Design review of the part built by this model. Coordinates are the model's own, in mm. Coordinates: 2 decimals unless noted, no trailing zeros. Loops run counter-clockwise (first coordinate to the right, second up) from the corner with the lowest first, then second, coordinate; pieces in that order, holes last.
Q1. Add section C-C on x = 11.5. Give the boundary of the cut face in (y, z).
Q2. Add section A-A on y = 0. Give the boundary of the cut face in (x, z) (3 decimals), and give its area (3 significant figures).
Q3. Wall thickness on probe 1 along X at (y, z) = (-23, -25) (3 decimals); probe 2 along Y at (x, z) = (2.45, -6.35); probe 3 along Z at (x, y) = (10, -8.5): over which ranges is each line inside the solid? List them lowest first.
Q4. Draft analysis for pull direction Z (two halves, no side actions). For faces 1 (the face through (7.871, 22.534, 11.721)), 2 (the face through (3.175, -7.8, -24.5)), 3 (the face through (1.565, 19.863, -19.846)), state which applies: released by +Z, released by -Z, zero draft, split by the parting line, or undercut.
Q5. For P1, Ø3, axis at y = -28.575, z = -6.35, coming from the +X side; P2, Ø4, axis at y = 8.79, z = -27.92, coming from the +X side (3 decimals); P3, Ø2, axis at x = 5.5, z = 20, coming from the -Y side; P4, Ø1.5, axis at x = 5, y = -11, coming from the +Z side, all flat-tipped, find the tip position at first contact; note any pin that passes through.
```python
from build123d import *

# Parameters (mm, degrees)
SKETCH2_R           = 37.5
SKETCH2_R_2         = 1.7272
SKETCH2_R_3         = 22.86
BOSS_EXTRUDE1_DEPTH = 3.175
SKETCH3_R           = 25.4
SKETCH3_R_2         = 22.86
BOSS_EXTRUDE2_DEPTH = 9.525


with BuildPart() as part:
    # Sketch2 → Boss-Extrude1 (new body)
    with BuildSketch(Plane(origin=(0, 0, 0), x_dir=(0, 0, -1), z_dir=(1, 0, 0))):
        Circle(SKETCH2_R)
        with Locations((27.921675913, 8.788238686)):
            Circle(SKETCH2_R_2, mode=Mode.SUBTRACT)
        with Locations((21.571675913, 19.786761314)):
            Circle(SKETCH2_R_2, mode=Mode.SUBTRACT)
        with Locations((-21.571675913, 19.786761314)):
            Circle(SKETCH2_R_2, mode=Mode.SUBTRACT)
        with Locations((-27.921675913, 8.788238686)):
            Circle(SKETCH2_R_2, mode=Mode.SUBTRACT)
        with Locations((-6.35, -28.575)):
            Circle(SKETCH2_R_2, mode=Mode.SUBTRACT)
        with Locations((6.35, -28.575)):
            Circle(SKETCH2_R_2, mode=Mode.SUBTRACT)
        Circle(SKETCH2_R_3, mode=Mode.SUBTRACT)
    extrude(amount=BOSS_EXTRUDE1_DEPTH)

    # Sketch3 → Boss-Extrude2 (add)
    with BuildSketch(Plane(origin=(3.175, 0, 0), x_dir=(0, 0, -1), z_dir=(1, 0, 0))):
        with Locations(Location((0, 0, 0), (0, 0, 180))):
            Circle(SKETCH3_R)
        Circle(SKETCH3_R_2, mode=Mode.SUBTRACT)
    extrude(amount=BOSS_EXTRUDE2_DEPTH)


solid = part.part
```
Entries:
1. outline: circle Ø50.8 at (0, 0); hole circle Ø45.72 at (0, 0)
2. outline: (0, -37.5) - (3.175, -37.5) - (3.175, -25.4) - (12.7, -25.4) - (12.7, -22.86) - (0, -22.86) - close; (0, 22.86) - (12.7, 22.86) - (12.7, 25.4) - (3.175, 25.4) - (3.175, 37.5) - (0, 37.5) - close
2. area: 141 mm2
3. probe 1: x = 0 to 3.175
3. probe 2: y = -36.96 to -30.3, -26.85 to -21.96, 21.96 to 36.96
3. probe 3: z = -23.94 to -21.22, 21.22 to 23.94
4. face 1: split by the parting line
4. face 2: zero draft
4. face 3: undercut
5. P1: passes through
5. P2: stops at x = 3.175
5. P3: stops at y = -16.86
5. P4: stops at z = 23.24
